Autodesk Inventor part; units mm, degrees
ref_plane "YZ Plane" through (0, 0, 0) normal (1, 0, 0) x (0, 1, 0)
ref_plane "XZ Plane" through (0, 0, 0) normal (0, 1, 0) x (-1, 0, 0)
ref_plane "XY Plane" through (0, 0, 0) normal (0, 0, 1) x (1, 0, 0)
sketch "Sketch1" plane through (0, 0, 0) normal (0, 0, 1) x (1, 0, 0)
  line L0 (0, 0) -> (12, 0)
  line L1 (12, 0) -> (12, 2.5)
  line L2 (12, 2.5) -> (4.8, 2.5)
  line L3 (4.8, 2.5) -> (4.3, 2.4)
  line L4 (4.3, 2.4) -> (3.8, 2.4)
  line L5 (3.5, 2.705) -> (2.7, 2.705)
  line L6 (2.7, 2.705) -> (0.755, 4.65)
  line L7 (0.755, 4.65) -> (0, 4.65)
  line L8 (0, 4.65) -> (0, 0)
  line L9 (3.5, 2.705) -> (3.5, 2.7)
  arc A0 (3.5, 2.7) -> (3.8, 2.4) centre (3.8, 2.7) ccw
  dimension "d17" = 12
  dimension "d18" = 0.755
  dimension "d19" = 2.7
  dimension "d20" = 0.8
  dimension "d21" = 9.3
  dimension "d22" = 5
  dimension "d23" = 4.8
  dimension "d25" = 45
  dimension "d26" = 0.5
  dimension "d28" = 0.3
  dimension "d29" = 7.2
  dimension "d30" = 0.3
  dimension "d52" = 2.1
revolve "Revolution1" add sketch "Sketch1" angle 360 about axis through (0, 0, 0) along (1, 0, 0)
thread "Thread1"
sketch "Sketch2" plane through (0, 0, 0) normal (-1, 0, 0) x (0, 0, 1)
  circle A0 centre (0, 0) radius 2.25 construction
  circle A1 centre (0, 0) radius 1.575 construction
  line L0 (0, 0) -> (1.364, 0.7875)
  line L1 (0, 0) -> (1.575, 0) construction
  line L2 (0, 0) -> (1.364, -0.7875)
  line L3 (0, 0) -> (1.575, 0) construction
  line L4 (1.364, 0.7875) -> (2.25, 0)
  line L5 (2.25, 0) -> (1.364, -0.7875)
  line L6 (-6.51, 0) -> (6.51, 0)
  dimension "d34" = 4.5
  dimension "d35" = 3.15
  dimension "d39" = 30
  dimension "d40" = 330
extrude "Extrusion1" cut sketch "Sketch2" against normal blind 1.51
pattern_circular "Circular Pattern1" count 6 over 360 about axis through (-10, 0, 0) along (1, 0, 0) of "Extrusion1"
fillet "Fillet1" radius 0.5 12 edges at (0.755, 0.7875, 1.364) (0.755, 0, 2.25) (0.755, -0.7875, 1.364) (0.755, -1.575, 0) (0.755, -1.9486, 1.125) (0.755, -1.9486, -1.125) (0.755, -0.7875, -1.364) (0.755, 0, -2.25) (0.755, 0.7875, -1.364) (0.755, 1.9486, -1.125) (0.755, 1.575, 0) (0.755, 1.9486, 1.125)
equation "\"d17\" = l_"
equation "\"d18\" = 0.5 * t"
equation "\"d19\" = k"
equation "\"d20\" = shldr"
equation "\"d21\" = dk"
equation "\"d22\" = d"
equation "\"d23\" = ds_"
equation "\"d25\" = 0.5 * headAngle"
equation "\"d26\" = x"
equation "\"d28\" = r"
equation "\"d29\" = b"
equation "\"d32\" = b"
equation "\"d34\" = A_"
equation "\"d35\" = 0.7 * A_"
equation "\"d43\" = t"
equation "\"d48\" = v"
equation "\"A_\" = 4.5"
equation "\"t\" = 1.51"
equation "\"v\" = 0.1 * d"
equation "\"dk\" = 9.3"
equation "\"k\" = 2.7"
equation "\"l_\" = 12"
equation "\"shldr\" = 0.8"
equation "\"d\" = 5"
equation "\"p\" = 0.8"
equation "\"x\" = 0.5"
equation "\"ds_\" = 0.96 * d"
equation "\"headAngle\" = 90deg"
equation "\"c_\" = 0.35 * v"
equation "\"r\" = 0.3"
properties part number "Senkkopfschraube mit Innenrund ISO 14581 - M5x12-4.8" material "Stahl"
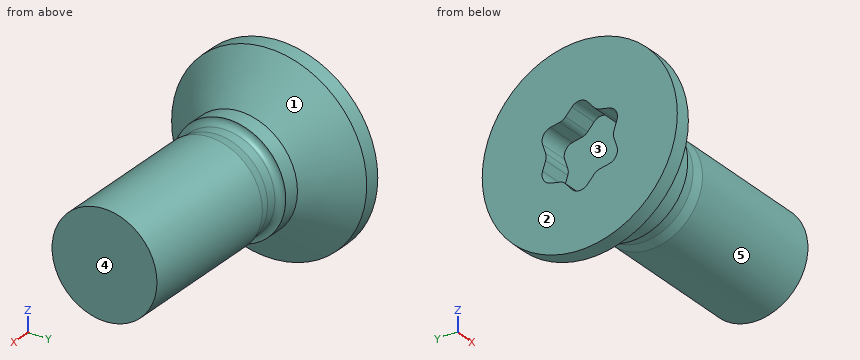
Design review of the part built by this model. Coordinates are the model's own, in mm. Face numbers are marked on the shaded views. A direction names the side the tool comes from. Round coordinates to 2 decimals unless told otherwise and drop trailing zeros. Write each loop counter-clockwise with the first axis right and the second up, starting at its lowest first coordinate (ties: lowest second). Pieces come first, ordered by that corner, then holes. Notation, with made-up numbers: (2.5, 23) -> (42.5, 23) arc R35 ccw to (42.5, 56) -> close; hole circle Ø2 at (-25, 75.25). An arc over 180 degrees is marked (long way). One line per item, written item: value. Start each with the question number.
Q1. Insertion check: P1, Ø5, axis at x = 3.5, y = -1, coming from the +Z side; P2, Ø1, axis at x = 2.5, y = -1.5, coming from the +Z side; P3, Ø1.5, axis at x = 4.5, y = 2, coming from the +Z side. Each pin has a flat end and moves straight along its axis. Give the tip position at first contact, or say it passes through.
Q2. The part is to be moulded in two halves that separate along Z. For the marked faces 1, 2 and 3, say which applies: pulls with the +Z half, pulls with the -Z half, needs draft (parallel to the pull), parting line crosses it, or undercut.
Q3. Tool access review of the marked faces 4 and 5: name each direction out of +Z, -Z, +X, -X, +Y, -Y from which nothing blocks a thin tool from reaching the whole face with its end or side.
Q4. Add section B-B (y = 0). Give the boundary of the cut face in (x, z) (3 decimals), then the cut area to 3 significant figures.
Q5. Add section A-A (z = 0). Give the boundary of the cut face in (x, y) (3 decimals).
Q6. Add section C-C (x = 7.5). Give the boundary of the cut face in (y, z), then the cut area to 3 significant figures.
Q7. Add section D-D (x = 2.5). Give the boundary of the cut face in (y, z) (3 decimals), then the cut area to 3 significant figures.
Q8. To check wall thickness, follow probe 1 along Y at (x, z) = (5.75, 1.5); probe 2 along X at (y, z) = (-1.75, 3.5); probe 3 along X at (y, z) = (-0.5, 1.5). State the ranges of each line that lie inside material, in increasing order.
Response:
1. P1: stops at z = 4.33
1. P2: stops at z = 3.1
1. P3: stops at z = 2.13
2. face 1: parting line crosses it
2. face 2: needs draft
2. face 3: undercut
3. face 4: +Z, -Z, +X, +Y, -Y
3. face 5: +X
4. outline: (0, -4.65) -> (0.755, -4.65) -> (2.7, -2.705) -> (3.5, -2.705) -> (3.5, -2.7) arc R0.3 cw to (3.8, -2.4) -> (4.3, -2.4) -> (4.8, -2.5) -> (12, -2.5) -> (12, 2.5) -> (4.8, 2.5) -> (4.3, 2.4) -> (3.8, 2.4) arc R0.3 cw to (3.5, 2.7) -> (3.5, 2.705) -> (2.7, 2.705) -> (0.755, 4.65) -> (0, 4.65) -> (0, 1.997) -> (1.51, 1.997) -> (1.51, -1.997) -> (0, -1.997) -> close
4. area: 62.0 mm^2
5. outline: (0, -4.65) -> (0.755, -4.65) -> (2.7, -2.705) -> (3.5, -2.705) -> (3.5, -2.7) arc R0.3 cw to (3.8, -2.4) -> (4.3, -2.4) -> (4.8, -2.5) -> (12, -2.5) -> (12, 2.5) -> (4.8, 2.5) -> (4.3, 2.4) -> (3.8, 2.4) arc R0.3 cw to (3.5, 2.7) -> (3.5, 2.705) -> (2.7, 2.705) -> (0.755, 4.65) -> (0, 4.65) -> (0, 1.602) -> (1.51, 1.602) -> (1.51, -1.602) -> (0, -1.602) -> close
6. outline: circle Ø5 at (0, 0)
6. area: 19.6 mm^2
7. outline: circle Ø5.81 at (0, 0)
7. area: 26.5 mm^2
8. probe 1: y = -2 to 2
8. probe 2: x = 0 to 1.49
8. probe 3: x = 1.51 to 12
